Build history of the part. All positions in model axes, mm. A direction names the side the tool comes from. Round coordinates to 2 decimals unless told otherwise and drop trailing zeros. Write each loop counter-clockwise with the first axis right and the second up, starting at its lowest first coordinate (ties: lowest second). Pieces come first, ordered by that corner, then holes. Notation, with made-up numbers: (11, 71) - (45, 71) arc R6 ccw to (45, 77) - close; hole circle Ø9 at (-38, 36). An arc over 180 degrees is marked (long way). Answer as a JSON object with one key per item and string values. Group by question number.
Item 1: Flat gauge pin, fed straight in: pin 1 (2 mm diameter, centred on y = -27, z = 3, fed in from +X). Where does the tip first touch, or does it go through?
Item 2: Probe line 1 (Y direction, x = 5, z = 0.55); line 2 (X direction, y = -15.5, z = 3.05); line 3 (X direction, y = 11, z = 1.15). List the from-to ranges inside material, lowest first. Write a range as from..to.
Item 3: Two-plate mould, pull along Y, no slides. Class faces 1 (the flat face through (-65, -5, 2)), 2 (the flat face through (-3, 20, 2)), 3 (the flat face through (-42.79, 9.92, 1.97)), 4 (the cylindrical face through (-64, -18, 2)): +Y half, -Y half, draft (parallel to the pull), parting line (faces both ways), or undercut.
Item 4: Slice it at B-B, the plane x = 7. List the corners of the cut face in (y, z).
Item 5: Slice it at A-A, the plane z = 2.4. List the corners of the cut face in (x, y), then the cut area to 3 significant figures.
Item 6: Slice it at C-C, the plane y = -25.5. List the corners of the cut face in (x, z), then the cut area to 3 significant figures.
Item 7: Which spindle directions (+Z, -Z, +X, -X, +Y, -Y) get a long thin tool onto all of the face, cutting with end or side? Do faces 5 (the flat face through (-34.097, 11.336, 1.972)), 6 (the flat face through (-38, -20, 2)), 7 (the flat face through (34, -20, 2)). Say none if no direction does.
Autodesk Inventor part; units mm, degrees
ref_plane "YZ Plane" through (0, 0, 0) normal (1, 0, 0) x (0, 1, 0)
ref_plane "XZ Plane" through (0, 0, 0) normal (0, 1, 0) x (-1, 0, 0)
ref_plane "XY Plane" through (0, 0, 0) normal (0, 0, 1) x (1, 0, 0)
sketch "Sketch3" plane through (0, 0, 0) normal (0, 0, 1) x (1, 0, 0)
  line L0 (-91, 0) -> (91, 0)
  line L1 (0, -48.6774) -> (0, 47.0644)
  line L2 (65, -10) -> (35, 20)
  line L3 (35, 20) -> (-31.6994, 20)
  line L4 (-31.6994, 20) -> (-36.1448, 3.9333)
  line L5 (65, -20) -> (2.5, -20)
  line L6 (2.5, -20) -> (2.5, -35)
  line L7 (2.5, -35) -> (-2.5, -35)
  line L8 (-2.5, -35) -> (-17.5, -20)
  line L9 (-17.5, -20) -> (-65, -20)
  line L10 (-65, -20) -> (-65, 20)
  line L11 (-65, 20) -> (-40, 20)
  line L12 (65, -20) -> (65, -10)
  line L13 (-40, 20) -> (-43.8552, 6.0667)
  arc A0 (-43.8552, 6.0667) -> (-36.1448, 3.9333) centre (-40, 5) ccw
  line L14 (-26.282, 1.2044) -> (-45.4203, 6.4997) construction
  line L15 (-40, -18.8457) -> (-40, 33.387) construction
  point P0 (0, 0)
  dimension "d0" = 130
  dimension "d1" = 40
  dimension "d2" = 10
  dimension "d4" = 5
  dimension "d5" = 20
  dimension "d6" = 30
  dimension "d8" = 55
  dimension "d11" = 8
  dimension "d12" = 25
  dimension "d16" = 8
  dimension "d23" = 15
extrude "Extrusion1" add sketch "Sketch3" along normal blind 4
fillet "Fillet1" radius 2 2 edges at (-31.6994, 20, 2) (65, -10, 2)
fillet "Fillet2" radius 30 1 edges at (35, 20, 2)
fillet "Fillet3" radius 5 2 edges at (-40, 20, 2) (-65, -20, 2)
fillet "Fillet4" radius 15 1 edges at (-65, 20, 2)
equation "\"BendRadius\" = Thickness"
equation "\"BendReliefWidth\" = Thickness"
equation "\"BendReliefDepth\" = 0.5 * Thickness"
equation "\"CornerReliefSize\" = 4 * Thickness"
equation "\"MinimumRemnant\" = 2 * Thickness"
equation "\"TransitionRadius\" = BendRadius"
equation "\"JacobiRadiusSize\" = BendRadius"
equation "\"GapSize\" = Thickness"
properties part number "Rear Wheel Holder"
Geometry says:
{
 "1": {"pin 1": "stops at x = 2.5"},
 "2": {"line 1": "y = -20..20", "line 2": "x = -64.97..65", "line 3": "x = -63.75..-42.49, -34.19..44"},
 "3": {"face 1": "draft", "face 2": "+Y half", "face 3": "undercut", "face 4": "-Y half"},
 "4": {"outline": "(-20, 0) - (20, 0) - (20, 4) - (-20, 4) - close"},
 "5": {"outline": "(-65, -15) arc R5 ccw to (-60, -20) - (-17.5, -20) - (-2.5, -35) - (2.5, -35) - (2.5, -20) - (65, -20) - (65, -10.83) arc R2 ccw to (64.41, -9.41) - (43.79, 11.21) arc R30 ccw to (22.57, 20) - (-30.18, 20) arc R2 ccw to (-32.11, 18.53) - (-36.14, 3.93) arc R4 cw to (-43.86, 6.07) - (-41.75, 13.67) arc R5 ccw to (-46.57, 20) - (-50, 20) arc R15 ccw to (-65, 5) - close", "area": "4,700 mm^2"},
 "6": {"outline": "(-12, 0) - (2.5, 0) - (2.5, 4) - (-12, 4) - close", "area": "58.0 mm^2"},
 "7": {"face 5": "+Z, -Z, +Y", "face 6": "+Z, -Z, -X, -Y", "face 7": "+Z, -Z, +X, -Y"}
}
